The model under review builds one solid part; all positions refer to its coordinate system, in mm. Face numbers are marked on the shaded views. A direction names the side the tool comes from. Coordinates: 2 decimals unless noted, no trailing zeros. Order: outer loops, then holes, each group sorted by start corner. A loop starts at its lowest first (then second) coordinate and runs counter-clockwise, first axis right, second up. Notation, with made-up numbers: M -7,53.5 L 17,53.5 A8 cw 17,59.5 Z; hole C 1.5,60.25 d3. An arc over 180 degrees is marked long. Answer as CSV lines item,"result". Start each with the question number.
Q1. Machinability: for the marked faces 4, 5, 6 and 7, which of the approach directions +Z, -Z, +X, -X, +Y, -Y give a long, thin tool a straight path to every point of the face, cutting with its end or side? Answer none if there is none.
Q2. Consider section D-D on z = -31. Write out the cut boundary in (x, y).
Q3. Consider section C-C on z = 33. Write out the cut boundary in (x, y), and give its area (3 significant figures).
Q4. Consider section B-B on x = -13. Write out the cut boundary in (y, z).
Q5. The part is to be moulded in two halves that separate along Y. For the marked faces 1, 2 and 3, say which applies: +Y half, -Y half, draft (parallel to the pull), parting line (faces both ways), or undercut.
Q6. For P1, Ø4, axis at x = 5.5, y = 11.5, coming from the +Z side; P2, Ø14.5, axis at x = -62, y = -10, coming from the +Z side; P3, Ø2, axis at x = 31, z = 43.5, coming from the -Y side; P4, Ø20, axis at y = -6.5, z = 64.5, coming from the +X side, all flat-tipped, find the tip position at first contact; note any pin that passes through.
Q7. Consider section A-A on y = -9.5. State how many separate pieces and enclosed holes the cut face has, and give its area (3 significant figures).
Q8. Wall thickness on L1, parallel to Z at x = 8.5, y = -12.5; L2, parallel to Z at x = 11, y = 15; L3, parallel to Y at x = -11, z = 48: over which ranges is each line inside the solid? List them lowest first. Write a range as [from, to].
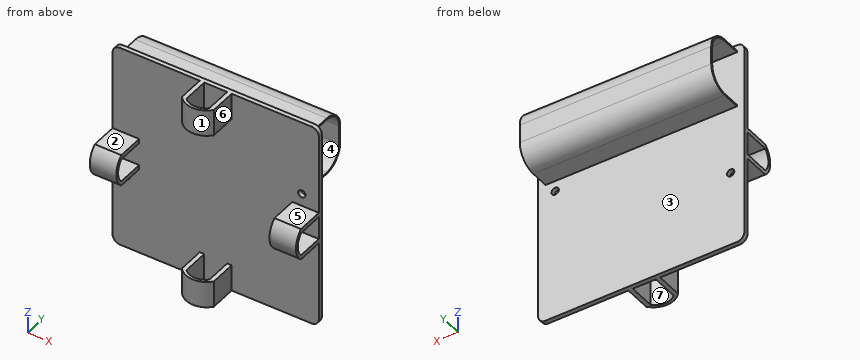
Autodesk Inventor part; units mm, degrees
ref_plane "Work Plane1" through (65, 0, 65) normal (1, 0, 0) x (0, 0, -1)
ref_plane "YZ Plane" through (0, 0, 0) normal (1, 0, 0) x (0, 1, 0)
ref_plane "XZ Plane" through (0, 0, 0) normal (0, 1, 0) x (-1, 0, 0)
sketch "Sketch1" plane through (0, 0, 0) normal (0, 1, 0) x (-1, 0, 0)
  line L0 (70, 0) -> (70, -70)
  line L1 (70, -70) -> (0, -70)
  line L2 (-70, 0) -> (-70, 70)
  line L3 (-70, 70) -> (0, 70)
  line L4 (0, 70) -> (70, 70)
  line L5 (70, 70) -> (70, 0)
  line L6 (0, -70) -> (-70, -70)
  line L7 (-70, -70) -> (-70, 0)
  point P0 (0, 0)
extrude "Extrusion1" add sketch "Sketch1" along normal blind 3
fillet "Fillet1" radius 5 3 edges at (70, 1.5, 70) (70, 1.5, -70) (-70, 1.5, 70)
fillet "Fillet2" radius 5 1 edges at (-70, 1.5, -70)
ref_plane "Work Plane1" through (65, 0, 65) normal (1, 0, 0) x (0, 0, -1)
sketch "Sketch5" plane through (65, 0, 65) normal (1, 0, 0) x (0, 0, -1)
  line L0 (0, 3) -> (0, 15.5)
  arc A0 (12.5, 28) -> (0, 15.5) centre (12.5, 15.5) ccw
  line L1 (12.5, 28) -> (25, 28)
  arc A1 (37.5, 15.5) -> (25, 28) centre (25, 15.5) ccw
  line L2 (37.5, 15.5) -> (37.5, 3)
  line L3 (0, 3) -> (130, 3)
  line L4 (0, 3) -> (-1, 3)
  line L5 (-5, 3) -> (0, 3)
  line L6 (-1, 3) -> (-1, 15.5)
  arc A2 (12.5, 29) -> (-1, 15.5) centre (12.5, 15.5) ccw
  line L7 (12.5, 29) -> (25, 29)
  arc A3 (38.5, 15.5) -> (25, 29) centre (25, 15.5) ccw
  line L8 (38.5, 15.5) -> (38.5, 3)
  line L9 (38.5, 3) -> (37.5, 3)
  line L10 (0, 3) -> (-1, 3)
  line L11 (0, 0) -> (0, 3)
  point P0 (65, 0)
  dimension "d9" = 12.5
  dimension "d11" = 12.5
  dimension "d12" = 1
extrude "Extrusion2" add sketch "Sketch5" against normal blind 130 contours L4 L6 A2 L7 A3 L8 L3 L2 A1 L1 A0 L0
sketch "Sketch6" plane through (70, 0, 65) normal (1, 0, 0) x (0, 0, -1)
  line L0 (65, 0) -> (57.2, 0)
  line L1 (130, 0) -> (0, 0)
  line L2 (65, 0) -> (72.8, 0)
  line L3 (57.2, 0) -> (57.2, -18)
  line L4 (72.8, 0) -> (72.8, -18)
  line L5 (65, 0) -> (65, -10)
  arc A0 (57.2, -18) -> (72.8, -18) centre (65, -10.2437) ccw
  line L6 (57.2, 0) -> (54.2, 0)
  line L7 (54.2, 0) -> (54.2, -18)
  line L8 (72.8, 0) -> (75.8, 0)
  line L9 (75.8, 0) -> (75.8, -18)
  arc A1 (54.2, -18) -> (75.8, -18) centre (65, -9.0916) ccw
  dimension "d17" = 18
  dimension "d21" = 3
  dimension "d22" = 3
extrude "Extrusion3" add sketch "Sketch6" against normal blind 18 contours L3 A0 L4 L1 L9 A1 L7
pattern_circular "Circular Pattern1" count 4 over 360 about axis through (0, -10, 0) along (0, 1, 0) of "Extrusion3"
sketch "Sketch8" plane through (0, 3, 0) normal (0, 1, 0) x (1, 0, 0)
  circle A0 centre (58.4636, -19.348) radius 2.5
  point P0 (0, 0)
  dimension "d35" = 5
extrude "Extrusion5" cut sketch "Sketch8" against normal blind 3
sketch "Sketch9" plane through (0, 3, 0) normal (0, 1, 0) x (1, 0, 0)
  circle A0 centre (-60.6489, 18.9578) radius 2.5
  point P0 (0, 0)
  dimension "d39" = 5
extrude "Extrusion6" cut sketch "Sketch9" against normal blind 3
properties part number "smallpart"
Evaluation:
1,face 4,"+X, -X"
1,face 5,"+Z, +X, -X, -Y"
1,face 6,"+Z, -Z, +X, -Y"
1,face 7,"+Z, -Z"
2,outline,"M -70,0 L 70,0 L 70,3 L -70,3 Z"
3,outline,"M -70,0 L 70,0 L 70,3 L -70,3 Z; M -65,25.86 L 65,25.86 L 65,27.04 L -65,27.04 Z"
3,area,"574 mm²"
4,outline,"M 0,-70 L 3,-70 L 3,26.5 L 15.5,26.5 A13.5 ccw 29,40 L 29,52.5 A13.5 ccw 15.5,66 L 3,66 L 3,70 L 0,70 Z; hole M 3,27.5 L 15.5,27.5 A12.5 ccw 28,40 L 28,52.5 A12.5 ccw 15.5,65 L 3,65 Z"
5,face 1,"-Y half"
5,face 2,"draft"
5,face 3,"undercut"
6,P1,"stops at z = 66"
6,P2,"stops at z = 10.8"
6,P3,"stops at y = 0"
6,P4,"stops at x = 70"
7,separate pieces,"8"
7,enclosed holes,"0"
7,area,"432 mm²"
8,L1,"z = [-70, -52], [52, 70]"
8,L2,"z = [26.5, 27.5], [65, 66]"
8,L3,"y = [0, 3], [28, 29]"
